```python
from build123d import *

# Parameters (mm, degrees)
F1_DEPTH     = 2
F2_W         = 1.7
F2_H         = 2
F2_W_2       = 6.3
F2_H_2       = 8
F3_DEPTH     = 1.3
F4_W         = 8
F4_H         = 10
F5_DEPTH     = 2
F6_R         = 5
F7_R         = 1
F8_T1_DEPTH  = 3.3
F8_T3_DEPTH  = 7.5
F8_T5_DEPTH  = 9.5
F8_T7_DEPTH  = 5.5
F8_T9_DEPTH  = 11.5
F8_S13_W     = 1
F8_S13_H     = 1
F8_T14_DEPTH = 1
F8_S19_W     = 1
F8_S19_H     = 1
F8_T20_DEPTH = 1
F8_T24_ANGLE = 90
F10_DEPTH    = 1.3


# Not quite as in the source:
# - a fillet or chamfer that OpenCascade refuses, or shapes differently, is made with other operations: its cross-section is extruded or revolved along the edge and cut away or added


with BuildPart() as f1:
    # F0 (on Top) → F1 (new body)
    with BuildSketch(Plane.XY):
        with BuildLine():
            Line((-6.5, -51), (6.5, -51))
            Line((6.5, -51), (6.5, 46))
            ThreePointArc((6.5, 46), (5.0355339059, 49.5355339059), (1.5, 51))
            Line((1.5, 51), (-6.5, 51))
            Line((-6.5, 51), (-6.5, -51))
        make_face()
    extrude(amount=F1_DEPTH)

    # F2 (on face) → F3 (join)
    with BuildSketch(Plane(origin=(0, 0, 0), x_dir=(1, 0, 0), z_dir=(0, 0, -1))):
        with Locations((-5.65, -50)):
            Rectangle(F2_W, F2_H)
        with Locations((-1.65, -50)):
            Rectangle(F2_W_2, F2_H)
        with Locations((-5.65, -45)):
            Rectangle(F2_W, F2_H_2)
    extrude(amount=F3_DEPTH)

    # F4 (on face) → F5 (join)
    with BuildSketch(Plane(origin=(0, 0, -1.3), x_dir=(1, 0, 0), z_dir=(0, 0, -1))):
        with Locations((-2.5, -46)):
            Rectangle(F4_W, F4_H)
    extrude(amount=F5_DEPTH)

    # F6
    f6_edges = [f1.edges().sort_by_distance(p)[0] for p in [
        (6.5, -51, 1),
        (1.5, 41, -2.3),
    ]]
    fillet(f6_edges, radius=F6_R)

    # F7
    f7_edges = [f1.edges().sort_by_distance(p)[0] for p in [
        (-2.5, -51, 2),
        (5.035534, -49.535534, 2),
        (-6.5, 0, 2),
        (6.5, 0, 2),
        (-2.5, 51, 2),
        (5.035534, 49.535534, 2),
    ]]
    fillet(f7_edges, radius=F7_R)

    # F8: fillet of radius 1 on 6 edges, made by hand

    # F8_s2 → F8_t1 (cut)
    with BuildSketch(Plane.XY.offset(-2.3)):
        with BuildLine():
            ThreePointArc((-5.5, 51), (-6.2071067812, 50.7071067812), (-6.5, 50))
            Line((-6.5, 50), (-6.5, 51))
            Line((-6.5, 51), (-5.5, 51))
        make_face()
    extrude(amount=F8_T1_DEPTH, mode=Mode.SUBTRACT)

    # F8_s4 → F8_t3 (cut)
    with BuildSketch(Plane.XZ.offset(-53.5)):
        with BuildLine():
            ThreePointArc((1.5, -2.3), (1.2071067812, -3.0071067812), (0.5, -3.3))
            Line((0.5, -3.3), (1.5, -3.3))
            Line((1.5, -3.3), (1.5, -2.3))
        make_face()
    extrude(amount=F8_T3_DEPTH, mode=Mode.SUBTRACT)

    # F8_s6 → F8_t5 (cut)
    with BuildSketch(Plane.YZ.offset(-5.5)):
        with BuildLine():
            ThreePointArc((51, -2.3), (50.7071067812, -3.0071067812), (50, -3.3))
            Line((50, -3.3), (51, -3.3))
            Line((51, -3.3), (51, -2.3))
        make_face()
    extrude(amount=F8_T5_DEPTH, mode=Mode.SUBTRACT)

    # F8_s8 → F8_t7 (cut)
    with BuildSketch(Plane.YZ.offset(-9)):
        with BuildLine():
            ThreePointArc((42, -3.3), (41.2928932188, -3.0071067812), (41, -2.3))
            Line((41, -2.3), (41, -3.3))
            Line((41, -3.3), (42, -3.3))
        make_face()
    extrude(amount=F8_T7_DEPTH, mode=Mode.SUBTRACT)

    # F8_s10 → F8_t9 (cut)
    with BuildSketch(Plane.XZ.offset(-50)):
        with BuildLine():
            ThreePointArc((-6.5, -2.3), (-6.2071067812, -3.0071067812), (-5.5, -3.3))
            Line((-5.5, -3.3), (-6.5, -3.3))
            Line((-6.5, -3.3), (-6.5, -2.3))
        make_face()
    extrude(amount=F8_T9_DEPTH, mode=Mode.SUBTRACT)


with BuildPart() as f8_tool12:
    # F8_s13 → F8_t14 (new body)
    with BuildSketch(Plane.XZ.offset(-50)):
        with Locations((-6, 1.5)):
            Rectangle(F8_S13_W, F8_S13_H)
    extrude(amount=-F8_T14_DEPTH)

    # F8_s15 → F8_t16 (revolve, cut)
    with BuildSketch(Plane(origin=(-5.5, 50, 1), x_dir=(0.7071067812, 0, -0.7071067812), z_dir=(0.7071067812, 0, 0.7071067812))):
        with BuildLine():
            ThreePointArc((0, -1), (1, 0), (0, 1))
            Line((0, 1), (0, -1))
        make_face()
    revolve(axis=Axis((-5.5, 50, 1), (0, 1, 0)), mode=Mode.SUBTRACT)


with BuildPart() as f1_1:
    add(f1.part)

    # F8_t11: cut F8_tool12
    add(f8_tool12.part, mode=Mode.SUBTRACT)


with BuildPart() as f8_tool18:
    # F8_s19 → F8_t20 (new body)
    with BuildSketch(Plane.XZ.offset(-50)):
        with Locations((-6, -2.8)):
            Rectangle(F8_S19_W, F8_S19_H)
    extrude(amount=-F8_T20_DEPTH)

    # F8_s21 → F8_t22 (revolve, cut)
    with BuildSketch(Plane(origin=(-5.5, 50, -2.3), x_dir=(0.7071067812, 0, 0.7071067812), z_dir=(-0.7071067812, 0, 0.7071067812))):
        with BuildLine():
            ThreePointArc((0, -1), (1, 0), (0, 1))
            Line((0, 1), (0, -1))
        make_face()
    revolve(axis=Axis((-5.5, 50, -2.3), (0, 1, 0)), mode=Mode.SUBTRACT)


with BuildPart() as f1_2:
    add(f1_1.part)

    # F8_t17: cut F8_tool18
    add(f8_tool18.part, mode=Mode.SUBTRACT)

    # F8_s23 → F8_t24 (revolve, cut)
    with BuildSketch(Plane.XZ.offset(-46)):
        with BuildLine():
            ThreePointArc((0.5, -3.3), (1.2071067812, -3.0071067812), (1.5, -2.3))
            Line((1.5, -2.3), (1.5, -3.3))
            Line((1.5, -3.3), (0.5, -3.3))
        make_face()
    revolve(axis=Axis((-3.5, 46, -3.3), (0, 0, -1)), revolution_arc=F8_T24_ANGLE, mode=Mode.SUBTRACT)

    # F9 (on face) → F10 (join, through all)
    with BuildSketch(Plane(origin=(0, 0, 0), x_dir=(1, 0, 0), z_dir=(0, 0, -1))):
        with BuildLine():
            ThreePointArc((-3.5, -42), (-0.6715728753, -43.1715728753), (0.5, -46))
            Line((0.5, -46), (1.5, -46))
            ThreePointArc((1.5, -46), (0.0355339059, -42.4644660941), (-3.5, -41))
            Line((-3.5, -41), (-3.5, -42))
        make_face()
    extrude(amount=F10_DEPTH)


solid = f1_2.part
```
Build history of the part. All positions in model axes, mm. A direction names the side the tool comes from. Give positions to 0.01 mm unless a question says otherwise; leave off trailing zeros. Loops run counter-clockwise (first coordinate to the right, second up) from the corner with the lowest first, then second, coordinate; pieces in that order, holes last. Notation, with made-up numbers: (48, 43.25) - (67, 43.25) arc R4 cw to (67, 48.25) - close; hole circle Ø5 at (22.25, 2.25). An arc over 180 degrees is marked (long way). Use a Markdown table: item, result.
(1) Which spindle directions (+Z, -Z, +X, -X, +Y, -Y) get a long thin tool onto all of the face, cutting with end or side? Do faces 5 (the face through (5.07, -49.5, 0.51)), 6 (the face through (1.5, 49, -2)). Say none if no direction does.
Taken from the geometry:
| item | result |
|---|---|
| face 5 | +Z, -Z, +X, -Y |
| face 6 | -Z, +X, +Y, -Y |
(2) Drop flat-ended pins along their axis: pin 1 Ø1.5 at (y, z) = (28, -2) entering from +X; pin 2 Ø1.8 at (y, z) = (47.5, -1) entering from +X; pin 3 Ø0.6 at (x, z) = (-2, -0.5) entering from -Y; pin 4 Ø1.2 at (x, z) = (-5, -1.5) entering from -Y. Give the stop position or say it passes through.
Taken from the geometry:
| item | result |
|---|---|
| pin 1 | through |
| pin 2 | x = 1.5 |
| pin 3 | y = 41.15 |
| pin 4 | y = 41 |
(3) Wall check: line 1 along Z through (x, y) = (-2, -2); line 2 along Y through (x, z) = (-4, -1.95); line 3 along X through (y, z) = (43.5, 1.2). Give the ranges that are in metal, low to high.
Taken from the geometry:
| item | result |
|---|---|
| line 1 | 0 to 2 |
| line 2 | 41 to 51 |
| line 3 | -6.48 to 6.48 |
(4) Band-saw the part on A-A (y = -5). Give the cut face in (x, z), and give its area (3 significant figures).
Taken from the geometry:
| item | result |
|---|---|
| outline | (-6.5, 0) - (6.5, 0) - (6.5, 1) arc R1 ccw to (5.5, 2) - (-5.5, 2) arc R1 ccw to (-6.5, 1) - close |
| area | 25.6 mm2 |
(5) Pull direction Y, two halves, no side cores. Call faces 1 (the face through (0, 1, 2)), 2 (the face through (-0.703, 43.141, -0.641)), 3 (the face through (-5, 41, -1)), 4 (the face through (-2, 46, -1.3)): +Y half, -Y half, draft (parallel to the pull), parting line (faces both ways), or undercut.
Taken from the geometry:
| item | result |
|---|---|
| face 1 | draft |
| face 2 | undercut |
| face 3 | -Y half |
| face 4 | undercut |
